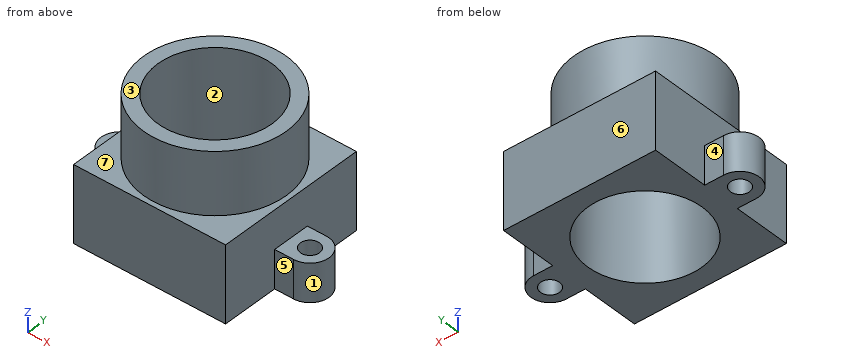
from build123d import *

# Parameters (mm, degrees)
F0_R     = 7.5
F0_R_2   = 6
F1_DEPTH = 14.5
F2_DEPTH = 8
F0_R_3   = 1
F3_DEPTH = 4


with BuildPart() as f1:
    # F0 (on Top) → F1 (new body)
    with BuildSketch(Plane.XY):
        Circle(F0_R)
        Circle(F0_R_2, mode=Mode.SUBTRACT)
    extrude(amount=F1_DEPTH)

    # F0 (on Top) → F2 (join)
    with BuildSketch(Plane.XY):
        Polygon((8, 2), (8, 8), (-8, 8), (-8, 2), (-8, -2), (-8, -8), (8, -8), (8, -2), align=None)
        Circle(F0_R, mode=Mode.SUBTRACT)
    extrude(amount=F2_DEPTH)

    # F0 (on Top) → F3 (join)
    with BuildSketch(Plane.XY):
        with BuildLine():
            Line((-8, -2), (-8, 2))
            Line((-8, 2), (-10, 2))
            ThreePointArc((-10, 2), (-12, 0), (-10, -2))
            Line((-10, -2), (-8, -2))
        make_face()
        with Locations((-10, 0)):
            Circle(F0_R_3, mode=Mode.SUBTRACT)
        with BuildLine():
            Line((10, 2), (8, 2))
            Line((8, 2), (8, -2))
            Line((8, -2), (10, -2))
            ThreePointArc((10, -2), (12, 0), (10, 2))
        make_face()
        with Locations((10, 0)):
            Circle(F0_R_3, mode=Mode.SUBTRACT)
    extrude(amount=F3_DEPTH)


solid = f1.part
Verification items for the finished model (mm, model axes). Face numbers are marked on the shaded views. A direction names the side the tool comes from. Give positions to 0.01 mm unless a question says otherwise; leave off trailing zeros. Write each loop counter-clockwise with the first axis right and the second up, starting at its lowest first coordinate (ties: lowest second). Pieces come first, ordered by that corner, then holes. Notation, with made-up numbers: M 40,81.5 L 98,81.5 A16 cw 98,109.5 Z; hole C 65.5,30 d2. An arc over 180 degrees is marked long. Put each result on its own line as item: value. Start each with the question number.
1. Section check D-D (z = 11.5). Record the cut outline in (x, y).
2. Set-up check for the marked faces 4, 5, 6 and 7: record each of +Z, -Z, +X, -X, +Y, -Y from which the full face is reachable in a straight line by a thin tool's end or side.
3. Section check C-C (y = 4). Record the cut outline in (x, z).
4. Section check B-B (x = 0). Record the cut outline in (y, z).
5. Section check A-A (y = 0). Record the cut outline in (x, z), and give its area (3 significant figures).
6. Go/stop test with flat-tipped pins: pin 1 Ø1.6 at (x, z) = (-9, 3) entering from +Y; pin 2 Ø3 at (x, y) = (-10.5, -0.5) entering from +Z; pin 3 Ø2.5 at (y, z) = (2.5, 5.5) entering from +X. Record where each tip stops, or that it passes through.
7. Draft check along Y on the marked faces 1, 2 and 3. Enter one of: +Y half, -Y half, draft (parallel to the pull), parting line (faces both ways), or undercut.
8. Scan lines: line 1 along Y through (x, z) = (10, 2); line 2 along Z through (x, y) = (6.25, -5.5); line 3 along Z through (x, y) = (8.5, 0.75). Record each from-to range of solid material in increasing order. Write a range as [from, to].
Answer list:
1. outline: C 0,0 d15; hole C 0,0 d12
2. face 4: +Z, -Z, -X, +Y
2. face 5: +Z, -Z, +X, -Y
2. face 6: +Z, -Z, +X, -X, +Y
2. face 7: +Z
3. outline: M -8,0 L -4.47,0 L -4.47,14.5 L -6.34,14.5 L -6.34,8 L -8,8 Z; M 4.47,0 L 8,0 L 8,8 L 6.34,8 L 6.34,14.5 L 4.47,14.5 Z
4. outline: M -8,0 L -6,0 L -6,14.5 L -7.5,14.5 L -7.5,8 L -8,8 Z; M 6,0 L 8,0 L 8,8 L 7.5,8 L 7.5,14.5 L 6,14.5 Z
5. outline: M -12,0 L -11,0 L -11,4 L -12,4 Z; M -9,0 L -6,0 L -6,14.5 L -7.5,14.5 L -7.5,8 L -8,8 L -8,4 L -9,4 Z; M 6,0 L 9,0 L 9,4 L 8,4 L 8,8 L 7.5,8 L 7.5,14.5 L 6,14.5 Z; M 11,0 L 12,0 L 12,4 L 11,4 Z
5. area: 67.5 mm2
6. pin 1: y = 2
6. pin 2: z = 4
6. pin 3: x = 8
7. face 1: parting line
7. face 2: undercut
7. face 3: draft
8. line 1: [-2, -1], [1, 2]
8. line 2: [0, 8]
8. line 3: [0, 4]
